For this review, take the finished solid that the model builds, in its own axes (mm). A direction names the side the tool comes from. Round coordinates to 2 decimals unless told otherwise and drop trailing zeros. Write each loop counter-clockwise with the first axis right and the second up, starting at its lowest first coordinate (ties: lowest second). Pieces come first, ordered by that corner, then holes. Notation, with made-up numbers: (-15.5, 55) -> (34.5, 55) arc R33 cw to (34.5, 88) -> close; hole circle Ø3 at (-36, -32.5). An arc over 180 degrees is marked (long way). Answer in a Markdown table with one row per item. Add a question column.
```python
from build123d import *

# Parameters (mm, degrees)
SKETCH1_R           = 1.5
BOSS_EXTRUDE1_DEPTH = 3
CUT_EXTRUDE1_DEPTH  = 3
SKETCH3_R           = 2.125
CUT_EXTRUDE3_DEPTH  = 4


with BuildPart() as part:
    # Sketch1 → Boss-Extrude1 (new body)
    with BuildSketch(Plane(origin=(0, 0, 0), x_dir=(0, 0, -1), z_dir=(1, 0, 0))):
        Polygon((13, 6.5), (17, 6.5), (17, -8.5), (13, -8.5), (13, -10), (-13, -10), (-13, -8.5), (-17, -8.5), (-17, 6.5), (-13, 6.5), (-13, 8), (13, 8), align=None)
        with Locations((-8.75, 0)):
            Circle(SKETCH1_R, mode=Mode.SUBTRACT)
        with Locations((8.75, 0)):
            Circle(SKETCH1_R, mode=Mode.SUBTRACT)
    extrude(amount=BOSS_EXTRUDE1_DEPTH)

    # Sketch2 → Cut-Extrude1 (cut)
    with BuildSketch(Plane(origin=(3, 0, 0), x_dir=(0, 0, -1), z_dir=(1, 0, 0))):
        with BuildLine():
            Line((-3, -10), (3, -10))
            ThreePointArc((3, -10), (0, -7), (-3, -10))
        make_face()
    extrude(amount=-CUT_EXTRUDE1_DEPTH, mode=Mode.SUBTRACT)

    # Sketch3 → Cut-Extrude3 (cut, through all)
    with BuildSketch(Plane(origin=(3, 0, 0), x_dir=(0, 0, -1), z_dir=(1, 0, 0))):
        with Locations((0, 0.641129032)):
            Circle(SKETCH3_R)
    extrude(amount=-CUT_EXTRUDE3_DEPTH, mode=Mode.SUBTRACT)


solid = part.part
```
1. We need section B-B (y = 2.25). Write out the cut boundary in (x, z), plus the area to 3 significant figures.
2. The part is to be moulded in two halves that separate along Z. For faces 1 (the flat face through (3, -3, 0)), 2 (the flat face through (1, 7, -13)), 3 (the flat face through (1, -1, 17)), 4 (the cylindrical face through (1.48, 0.07, 10.25)), say which applies: pulls with the +Z half, pulls with the -Z half, needs draft (parallel to the pull), parting line crosses it, or undercut.
3. Tool access review of faces 5 (the flat face through (1, 6.5, 15)), 6 (the flat face through (1, -9, -13)), 7 (the flat face through (1, 6.5, -15)), 8 (the flat face through (1, -8.5, 15)), 9 (the flat face through (1, -10, -8)): name each direction out of +Z, -Z, +X, -X, +Y, -Y from which nothing blocks a thin tool from reaching the whole face with its end or side.
4. For L1, parallel to Z at x = 1.6, y = 0.5; L2, parallel to Z at x = 0.75, y = -0.25; L3, parallel to Y at x = 0.85, z = 0, list the stretches that pass through material, from the lowest coordinate up. Write a range as [from, to].
5. We need section A-A (z = 0). Write out the cut boundary in (x, y), plus the area to 4 significant figures.
6. Clearance check with flat-ended pins moving along their axes: pin 1 Ø1.2 at (x, y) = (1, 7.5) entering from -Z; pin 2 Ø0.9 at (x, z) = (2, -14) entering from -Y; pin 3 Ø1.2 at (x, y) = (2, 7.5) entering from +Z. State where each tip first meets the part, or that it passes through.
7. We need section C-C (x = 0.45). Write out the cut boundary in (y, z) (3 decimals).
Response:
| question | item | result |
|---|---|---|
| 1 | outline | (0, -17) -> (3, -17) -> (3, -1.39) -> (0, -1.39) -> close; (0, 1.39) -> (3, 1.39) -> (3, 17) -> (0, 17) -> close |
| 1 | area | 93.7 mm2 |
| 2 | face 1 | needs draft |
| 2 | face 2 | pulls with the -Z half |
| 2 | face 3 | pulls with the +Z half |
| 2 | face 4 | undercut |
| 3 | face 5 | +Z, +X, -X, +Y |
| 3 | face 6 | -Z, +X, -X, -Y |
| 3 | face 7 | -Z, +X, -X, +Y |
| 3 | face 8 | +Z, +X, -X, -Y |
| 3 | face 9 | +Z, -Z, +X, -X, -Y |
| 4 | L1 | [-17, -10.16], [-7.34, -2.12], [2.12, 7.34], [10.16, 17] |
| 4 | L2 | [-17, -10.23], [-7.27, -1.93], [1.93, 7.27], [10.23, 17] |
| 4 | L3 | [-7, -1.48], [2.77, 8] |
| 5 | outline | (0, -7) -> (3, -7) -> (3, -1.48) -> (0, -1.48) -> close; (0, 2.77) -> (3, 2.77) -> (3, 8) -> (0, 8) -> close |
| 5 | area | 32.25 mm2 |
| 6 | pin 1 | z = -13 |
| 6 | pin 2 | y = -8.5 |
| 6 | pin 3 | z = 13 |
| 7 | outline | (-10, -13) -> (-8.5, -13) -> (-8.5, -17) -> (6.5, -17) -> (6.5, -13) -> (8, -13) -> (8, 13) -> (6.5, 13) -> (6.5, 17) -> (-8.5, 17) -> (-8.5, 13) -> (-10, 13) -> (-10, 3) arc R3 cw to (-10, -3) -> close; hole circle Ø3 at (0, -8.75); hole circle Ø3 at (0, 8.75); hole circle Ø4.25 at (0.641, 0) |
